Could you check a few things on this model? Use its own coordinates, in mm. Coordinates: 2 decimals unless noted, no trailing zeros. Order: outer loops, then holes, each group sorted by start corner. A loop starts at its lowest first (then second) coordinate and runs counter-clockwise, first axis right, second up. Notation, with made-up numbers: (14.25, 28) - (61.25, 28) arc R24 cw to (61.25, 63) - close; hole circle Ø7 at (82, -12.75). An arc over 180 degrees is marked (long way). Answer as CSV lines item,"result". Start each with the question number.
1. I want a section at A-A, the plane y = 5.25. List the corners of the cut face in (x, z) for me.
2. I need wall thicknesses on probe 1 along X at (y, z) = (10.25, 0.5); probe 2 along Y at (x, z) = (20.25, 1.5); probe 3 along Y at (x, z) = (15.75, 0.5). Which ranges of each line are inside material? Lowest first, please.
3. I want a section at B-B, the plane x = 7.5. List the corners of the cut face in (y, z) for me.
4. I want a section at C-C, the plane z = 0.6. List the corners of the cut face in (x, y) for me, and give its area (3 significant figures).
from build123d import *

# Parameters (mm, degrees)
SKETCH_W        = 25
SKETCH_H        = 25
PAD_DEPTH       = 2.5
CHAMFER_SIZE    = 2
CHAMFER001_SIZE = 1.5
CHAMFER002_SIZE = 1


with BuildPart() as part:
    # Sketch → Pad (new body)
    with BuildSketch(Plane.XY):
        with Locations((12.5, 12.5)):
            Rectangle(SKETCH_W, SKETCH_H)
    extrude(amount=PAD_DEPTH)

    # Chamfer
    chamfer_edges = [part.edges().sort_by_distance(p)[0] for p in [
        (12.5, 0, 0),
    ]]
    chamfer(chamfer_edges, length=CHAMFER_SIZE)

    # Chamfer001
    chamfer001_edges = [part.edges().sort_by_distance(p)[0] for p in [
        (25, 13.5, 0),
    ]]
    chamfer(chamfer001_edges, length=CHAMFER001_SIZE)

    # Chamfer002
    chamfer002_edges = [part.edges().sort_by_distance(p)[0] for p in [
        (11.75, 25, 0),
    ]]
    chamfer(chamfer002_edges, length=CHAMFER002_SIZE)


solid = part.part
Solved:
1,outline,"(0, 0) - (23.5, 0) - (25, 1.5) - (25, 2.5) - (0, 2.5) - close"
2,probe 1,"x = 0 to 24"
2,probe 2,"y = 0.5 to 25"
2,probe 3,"y = 1.5 to 24.5"
3,outline,"(0, 2) - (2, 0) - (24, 0) - (25, 1) - (25, 2.5) - (0, 2.5) - close"
4,outline,"(0, 1.4) - (24.1, 1.4) - (24.1, 24.6) - (0, 24.6) - close"
4,area,"559 mm2"
